Geometry check sheet. Reference: the model listing, model coordinates, mm. Face numbers are marked on the shaded views. Give positions to 0.01 mm unless a question says otherwise; leave off trailing zeros. Loops run counter-clockwise (first coordinate to the right, second up) from the corner with the lowest first, then second, coordinate; pieces in that order, holes last.
1. Material ranges on L1, parallel to Z at x = 3, y = 0; L2, parallel to Z at x = 5.65, y = 0 (3 decimals); L3, parallel to Z at x = 11.5, y = -2, recorded low to high.
2. Release check for a two-part mould opening along Z. For the marked faces 1, 2, 3 and 4 record: +Z half, -Z half, draft (parallel to the pull), parting line (faces both ways), or undercut.
3. Go/stop test with flat-tipped pins: pin 1 Ø3 at (x, z) = (19.5, -73) entering from +Y; pin 2 Ø5 at (y, z) = (0, 0) entering from +X; pin 3 Ø3.5 at (y, z) = (0, -101.9) entering from -X; pin 4 Ø19 at (y, z) = (-13, -62.5) entering from +X. Record where each tip stops, or that it passes through.
4. Cross-section at D-D, the plane z = -37. Record the cut outline in (x, y).
5. Cross-section at A-A, the plane z = 0. Record the cut outline in (x, y) (3 decimals), plus the area to 3 significant figures.
6. Cross-section at C-C, the plane x = 16.5. Record the cut outline in (y, z).
7. Cross-section at B-B, the plane y = 0. Record the cut outline in (x, z) (3 decimals).
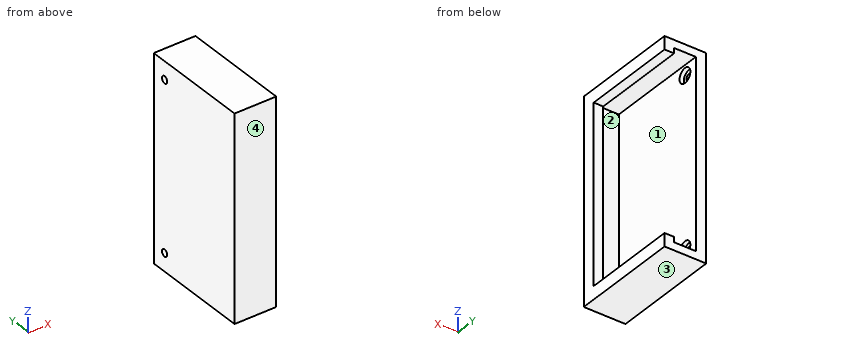
Autodesk Inventor part; units mm, degrees
ref_plane "YZ Plane" through (0, 0, 0) normal (1, 0, 0) x (0, 1, 0)
ref_plane "XZ Plane" through (0, 0, 0) normal (0, 1, 0) x (-1, 0, 0)
ref_plane "XY Plane" through (0, 0, 0) normal (0, 0, 1) x (1, 0, 0)
sketch "Sketch1" plane through (0, 0, 0) normal (1, 0, 0) x (0, 1, 0)
  circle A0 centre (0, 0) radius 3.9624 construction
  line L0 (3.9624, 0) -> (8.9624, 0) construction
  line L1 (0, 3.9624) -> (0, 10.9624) construction
  circle A1 centre (0, -101.9002) radius 3.9624 construction
  line L2 (3.9624, -101.9002) -> (8.9624, -101.9002) construction
  line L3 (0, -105.8626) -> (0, -112.8626) construction
  line L4 (8.9624, -112.8626) -> (-57.7126, -112.8626)
  line L5 (-57.7126, -112.8626) -> (-57.7126, 10.9624)
  line L6 (-57.7126, 10.9624) -> (8.9624, 10.9624)
  line L7 (8.9624, 10.9624) -> (8.9624, -112.8626)
  dimension "d0" = 7.9248
  dimension "d1" = 5
  dimension "d13" = 7
  dimension "d15" = 7.9248
  dimension "d16" = 5
  dimension "d17" = 7
extrude "Back plate" add sketch "Sketch1" along normal blind 6.35
sketch "Sketch5" plane through (6.35, 0, 0) normal (1, 0, 0) x (0, 0, -1)
  circle A0 centre (101.9002, 0) radius 3.9624
  circle A1 centre (0, 0) radius 3.9624
hole "Screw holes" at (6.35, 0, 0) at (6.35, 0, -101.9002) direction (-1, 0, 0) diameter 4.318 end through all counterbore diameter 8.89 counterbore depth 2.54
sketch "Sketch3" plane through (6.35, 0, 0) normal (1, 0, 0) x (0, 0, -1)
  line L0 (-10.9624, 8.9624) -> (-6.1999, 8.9624) construction
  line L1 (-10.9624, 8.9624) -> (-10.9624, -57.7126)
  line L2 (-6.1999, 8.9624) -> (-10.9624, 8.9624)
  line L3 (-10.9624, 8.9624) -> (-10.9624, -57.7126)
  line L4 (-10.9624, -57.7126) -> (-6.1999, -57.7126)
  line L5 (-6.1999, -57.7126) -> (-6.1999, 8.9624)
  line L6 (112.8626, -57.7126) -> (112.8626, 8.9624)
  line L7 (112.8626, 8.9624) -> (108.1001, 8.9624) construction
  line L8 (108.1001, 8.9624) -> (112.8626, 8.9624)
  line L9 (112.8626, 8.9624) -> (112.8626, -57.7126)
  line L10 (112.8626, -57.7126) -> (108.1001, -57.7126)
  line L11 (108.1001, -57.7126) -> (108.1001, 8.9624)
  line L12 (-6.1999, -54.5376) -> (108.1001, -54.5376)
  line L13 (108.1001, -54.5376) -> (108.1001, -57.7126)
  line L14 (108.1001, -57.7126) -> (-6.1999, -57.7126)
  point P0 (0, 0)
  point P1 (112.8626, 8.9624)
  dimension "d21" = 4.7625
  dimension "d22" = 4.7625
  dimension "d23" = 3.175
extrude "Sides and bottom" add sketch "Sketch3" along normal blind 19.05
sketch "Sketch4" plane through (6.35, -54.5376, 6.1999) normal (0, 0, -1) x (-1, 0, 0)
  line L0 (0, 63.5) -> (-19.05, 63.5) construction
  line L1 (0, 0) -> (-19.05, 0)
  line L2 (-19.05, 0) -> (-13.208, 0)
  line L3 (-13.208, 0) -> (-13.208, 63.5)
  line L4 (-13.208, 63.5) -> (-19.05, 63.5)
  line L5 (-19.05, 63.5) -> (-19.05, 0)
  point P0 (6.35, 54.5376)
  dimension "d28" = 5.842
extrude "Left lip" add sketch "Sketch4" along normal blind 3.175
sketch "Sketch6" plane through (6.35, -54.5376, -108.1001) normal (0, 0, 1) x (1, 0, 0)
  line L0 (19.05, 63.5) -> (19.05, 0) construction
  line L1 (19.05, 63.5) -> (13.208, 63.5) construction
  line L2 (0, 63.5) -> (19.05, 63.5) construction
  line L3 (19.05, 0) -> (13.208, 0)
  line L4 (13.208, 0) -> (13.208, 63.5)
  line L5 (13.208, 63.5) -> (19.05, 63.5)
  line L6 (19.05, 63.5) -> (19.05, 0)
  point P0 (-6.35, 54.5376)
  dimension "d38" = 5.842
extrude "Right lip" add sketch "Sketch6" along normal blind 3.175
sketch "Sketch7" plane through (6.35, -54.5376, 6.1999) normal (0, 1, 0) x (1, 0, 0)
  line L0 (13.208, 0) -> (13.208, 3.175)
  line L1 (13.208, 3.175) -> (19.05, 3.175)
  line L2 (19.05, 3.175) -> (19.05, 111.125)
  line L3 (19.05, 111.125) -> (13.208, 111.125)
  line L4 (13.208, 111.125) -> (13.208, 3.175)
  point P0 (-6.35, 6.1999)
extrude "Bottom lip" add sketch "Sketch7" along normal blind 5
properties part number "License Plate Holder"
Result:
1. L1: z = -112.86 to -104.06, -99.74 to -2.16, 2.16 to 10.96
1. L2: z = -112.863 to -106.345, -97.455 to -4.445, 4.445 to 10.962
1. L3: z = -112.86 to -108.1, 6.2 to 10.96
2. face 1: undercut
2. face 2: undercut
2. face 3: -Z half
2. face 4: draft
3. pin 1: stops at y = -49.54
3. pin 2: stops at x = 3.81
3. pin 3: passes through
3. pin 4: stops at x = 6.35
4. outline: (0, -57.71) - (25.4, -57.71) - (25.4, -49.54) - (19.56, -49.54) - (19.56, -54.54) - (6.35, -54.54) - (6.35, 8.96) - (0, 8.96) - close
5. outline: (0, -57.713) - (25.4, -57.713) - (25.4, -49.538) - (19.558, -49.538) - (19.558, -54.538) - (6.35, -54.538) - (6.35, -4.445) - (3.81, -4.445) - (3.81, -2.159) - (0, -2.159) - close; (0, 2.159) - (3.81, 2.159) - (3.81, 4.445) - (6.35, 4.445) - (6.35, 8.962) - (0, 8.962) - close
5. area: 474 mm2
6. outline: (-57.71, -112.86) - (8.96, -112.86) - (8.96, -108.1) - (-54.54, -108.1) - (-54.54, 6.2) - (8.96, 6.2) - (8.96, 10.96) - (-57.71, 10.96) - close
7. outline: (0, -112.863) - (25.4, -112.863) - (25.4, -104.925) - (19.558, -104.925) - (19.558, -108.1) - (6.35, -108.1) - (6.35, -106.345) - (3.81, -106.345) - (3.81, -104.059) - (0, -104.059) - close; (0, -99.741) - (3.81, -99.741) - (3.81, -97.455) - (6.35, -97.455) - (6.35, -4.445) - (3.81, -4.445) - (3.81, -2.159) - (0, -2.159) - close; (0, 2.159) - (3.81, 2.159) - (3.81, 4.445) - (6.35, 4.445) - (6.35, 6.2) - (19.558, 6.2) - (19.558, 3.025) - (25.4, 3.025) - (25.4, 10.962) - (0, 10.962) - close
